Here's how the part is built. I have some questions about the finished solid (model axes, mm). Face numbers are marked on the shaded views. A direction names the side the tool comes from. Coordinates: 2 decimals unless noted, no trailing zeros. Write each loop counter-clockwise with the first axis right and the second up, starting at its lowest first coordinate (ties: lowest second). Pieces come first, ordered by that corner, then holes.
(1) Please list where these lines run through material, in increasing order: probe 1 along Z at (x, y) = (20, -109); probe 2 along Y at (x, z) = (14, 14); probe 3 along Y at (x, z) = (19.25, 14).
(2) Thinking about a two-plate mould opening in Y: for the marked faces 4, 5 and 6, which applies, released by +Y, released by -Y, zero draft, split by the parting line, or undercut?
(3) Imagine slicing it at B-B, the plane y = -109.7. List the corners of the cut face in (x, z) for me.
(4) Imagine slicing it at C-C, the plane x = 114.5. List the corners of the cut face in (y, z) for me.
(5) For pin 1 Ø5 at (x, z) = (146, 25) entering from +Y; pin 2 Ø5 at (x, z) = (71, 8) entering from -Y; pin 3 Ø6 at (x, z) = (124.5, 18) entering from -Y; pin 4 Ø7 at (y, z) = (-109.7, 14) entering from +X, each with a flat end and sliding along its axis, tell me the tip position at first contact or that it passes through.
(6) Which directions (+Z, -Z, +X, -X, +Y, -Y) give clear straight access to the entire face, cutting with the end or side of a thin tool? Please do the marked faces 1, 2 and 3.
(7) Imagine slicing it at D-D, the plane y = 53.5. List the corners of the cut face in (x, z) for me.
(8) Imagine slicing it at A-A, the plane z = 14. List the corners of the cut face in (x, y) for me.
```python
from build123d import *

# Parameters (mm, degrees)
SKETCH1_R           = 8
BOSS_EXTRUDE1_DEPTH = 28
SKETCH2_R           = 6
CUT_EXTRUDE1_DEPTH  = 28


with BuildPart() as part:
    # Sketch1 → Boss-Extrude1 (new body)
    with BuildSketch(Plane.XY):
        with BuildLine():
            Line((0, -122), (0, -80.5))
            ThreePointArc((0, -80.5), (80.5, 0), (0, 80.5))
            Line((0, 80.5), (0, 122))
            Line((0, 122), (25, 122))
            Line((25, 122), (25, 97.340895825))
            ThreePointArc((25, 97.340895825), (52.885741133, 85.459630146), (75.960679556, 65.804446365))
            ThreePointArc((75.960679556, 65.804446365), (125.062415213, 29.040494844), (185, 16))
            Line((185, 16), (215, 16))
            ThreePointArc((215, 16), (231, 0), (215, -16))
            Line((215, -16), (185, -16))
            ThreePointArc((185, -16), (125.062415213, -29.040494844), (75.960679556, -65.804446365))
            ThreePointArc((75.960679556, -65.804446365), (52.885741133, -85.459630146), (25, -97.340895825))
            Line((25, -97.340895825), (25, -122))
            Line((25, -122), (0, -122))
        make_face()
        with Locations((215, 0)):
            Circle(SKETCH1_R, mode=Mode.SUBTRACT)
    extrude(amount=BOSS_EXTRUDE1_DEPTH)

    # Sketch2 → Cut-Extrude1 (cut)
    with BuildSketch(Plane.ZY):
        with Locations((14, 109.7)):
            Circle(SKETCH2_R)
        with Locations((14, -109.7)):
            Circle(SKETCH2_R)
    extrude(amount=-CUT_EXTRUDE1_DEPTH, mode=Mode.SUBTRACT)


solid = part.part
```
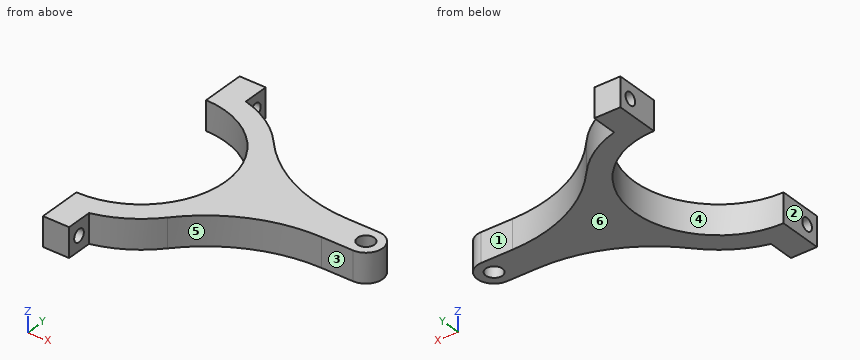
Recorded:
1. probe 1: z = 0 to 8.04, 19.96 to 28
1. probe 2: y = -122 to -115.7, -103.7 to -79.27, 79.27 to 103.7, 115.7 to 122
1. probe 3: y = -122 to -115.7, -103.7 to -78.16, 78.16 to 103.7, 115.7 to 122
2. face 4: undercut
2. face 5: released by -Y
2. face 6: zero draft
3. outline: (0, 0) - (25, 0) - (25, 8) - (0, 8) - close; (0, 20) - (25, 20) - (25, 28) - (0, 28) - close
4. outline: (-34.4, 0) - (34.4, 0) - (34.4, 28) - (-34.4, 28) - close
5. pin 1: stops at y = 22.1
5. pin 2: stops at y = -73.54
5. pin 3: stops at y = -30.73
5. pin 4: passes through
6. face 1: +Z, -Z, +X, +Y
6. face 2: +Z, -Z, -X, +Y, -Y
6. face 3: +Z, -Z, +X, -Y
7. outline: (60.15, 0) - (87.98, 0) - (87.98, 28) - (60.15, 28) - close
8. outline: (0, -122) - (25, -122) - (25, -115.7) - (0, -115.7) - close; (0, -103.7) - (25, -103.7) - (25, -97.34) arc R100.5 ccw to (75.96, -65.8) arc R144.26 cw to (185, -16) - (215, -16) arc R16 ccw to (215, 16) - (185, 16) arc R144.26 cw to (75.96, 65.8) arc R100.5 ccw to (25, 97.34) - (25, 103.7) - (0, 103.7) - (0, 80.5) arc R80.5 cw to (0, -80.5) - close; (0, 115.7) - (25, 115.7) - (25, 122) - (0, 122) - close; hole circle Ø16 at (215, 0)
